Autodesk Inventor part; units mm, degrees
ref_plane "YZ Plane" through (0, 0, 0) normal (1, 0, 0) x (0, 1, 0)
ref_plane "XZ Plane" through (0, 0, 0) normal (0, 1, 0) x (-1, 0, 0)
ref_plane "XY Plane" through (0, 0, 0) normal (0, 0, 1) x (1, 0, 0)
sketch "Sketch1" plane through (0, 0, 0) normal (0, 1, 0) x (-1, 0, 0)
  circle A0 centre (0, 0) radius 285
  circle A1 centre (0, 0) radius 295
  circle A2 centre (0, 0) radius 275
  circle A3 centre (0, 0) radius 305
  line L0 (0, 0) -> (300.3664, -52.9627)
  line L1 (0, 0) -> (305, 0)
  point P0 (275, 0)
  point P1 (270.8221, -47.7532)
  dimension "d1" = 590
  dimension "d5" = 10
  dimension "d6" = 10
  dimension "d7" = 10
  dimension "d8" = 10
extrude "Extrusion1" add sketch "Sketch1" along normal blind 10 contours L1 A1 L0 A0 | A0 L0 A2 L1 | L1 A3 L0 A1 picked at (291.5003, -5.7176) picked at (281.3509, -10.8537) picked at (297.9408, -46.5324)
sketch "Sketch2" plane through (0, 10, 0) normal (0, 1, 0) x (1, 0, 0)
  arc A0 (-270.8221, 47.7532) -> (-275, 0) centre (0, 0) ccw
  line L0 (-270.8221, 47.7532) -> (-300.3664, 52.9627)
  arc A1 (-300.3664, 52.9627) -> (-305, 0) centre (0, 0) ccw
  line L1 (-305, 0) -> (-275, 0)
  circle A2 centre (0, 0) radius 295
  circle A3 centre (0, 0) radius 285
  point P0 (-285, 0)
  point P1 (-280.6702, 49.4897)
  point P2 (-290.5183, 51.2262)
  point P3 (-295, 0)
  dimension "d11" = 10
  dimension "d12" = 590
extrude "Extrusion2" add sketch "Sketch2" along normal blind 5 contours A3 L1 A2 L0 picked at (-291.3396, 11.2413)
sketch "Sketch3" plane through (0, 15, 0) normal (0, 1, 0) x (1, 0, 0)
  line L0 (-290.5183, 51.2262) -> (-300.3664, 52.9627)
  arc A0 (-300.3664, 52.9627) -> (-305, 0) centre (0, 0) ccw
  line L1 (-305, 0) -> (-295, 0)
  line L2 (-280.6702, 49.4897) -> (-290.5183, 51.2262)
  arc A1 (-290.5183, 51.2262) -> (-295, 0) centre (0, 0) ccw
  line L3 (-295, 0) -> (-285, 0)
  arc A2 (-280.6702, 49.4897) -> (-285, 0) centre (0, 0) ccw
  line L4 (-285, 0) -> (-275, 0)
  arc A3 (-270.8221, 47.7532) -> (-275, 0) centre (0, 0) ccw
  line L5 (-270.8221, 47.7532) -> (-280.6702, 49.4897)
  circle A4 centre (0, 0) radius 305
  circle A5 centre (0, 0) radius 275
  line L6 (0, 0) -> (-304.7097, -13.3039)
  line L7 (0, 0) -> (-297.7703, 66.0141)
  arc A6 (-300.3664, 52.9627) -> (-305, 0) centre (0, 0) ccw
  arc A7 (-270.8221, 47.7532) -> (-275, 0) centre (0, 0) ccw
  arc A8 (-290.5183, 51.2262) -> (-295, 0) centre (0, 0) ccw
  line L8 (-290.5183, 51.2262) -> (-300.3664, 52.9627)
  line L9 (-305, 0) -> (-295, 0)
  arc A9 (-280.6702, 49.4897) -> (-285, 0) centre (0, 0) ccw
  arc A10 (-290.5183, 51.2262) -> (-295, 0) centre (0, 0) ccw
  arc A11 (-280.6702, 49.4897) -> (-285, 0) centre (0, 0) ccw
  line L10 (-285, 0) -> (-275, 0)
  line L11 (-270.8221, 47.7532) -> (-280.6702, 49.4897)
  point P0 (-270.8221, 47.7532)
  point P1 (-268.4814, 59.5209)
  point P2 (-305, 0)
  point P3 (-274.7383, -11.9953)
  point P4 (-305, 0)
  point P5 (-300.3664, 52.9627)
  point P6 (-305, 0)
  point P7 (-270.8221, 47.7532)
  dimension "d23" = 2.5
  dimension "d24" = 2.5
extrude "Extrusion3" add sketch "Sketch3" along normal blind 10 contours A1 L1 A0 L0 | L0 A4 L7 A5 L5 L2 | L2 A2 L3 A1 | L5 A3 L4 A2 | L3 L4 A5 L6 A4 L1
sketch "Sketch4" plane through (0, 0, 0) normal (0, -1, 0) x (1, 0, 0)
  arc A0 (-275, 0) -> (-270.8221, -47.7532) centre (0, 0) ccw
  line L0 (-305, 0) -> (-275, 0)
  arc A1 (-305, 0) -> (-300.3664, -52.9627) centre (0, 0) ccw
  line L1 (-270.8221, -47.7532) -> (-300.3664, -52.9627)
  circle A2 centre (0, 0) radius 285
  circle A3 centre (0, 0) radius 295
  point P0 (-295, 0)
  point P1 (-290.5183, -51.2262)
  point P2 (-280.6702, -49.4897)
  point P3 (-285, 0)
  dimension "d17" = 10
  dimension "d18" = 590
extrude "Extrusion4" add sketch "Sketch4" along normal blind 30 contours A2 L1 A3 L0 picked at (-291.3396, -11.2413)
sketch "Sketch5" plane through (0, -30, 0) normal (0, -1, 0) x (1, 0, 0)
  arc A0 (-295, 0) -> (-290.5183, -51.2262) centre (0, 0) ccw
  line L0 (-290.5183, -51.2262) -> (-280.6702, -49.4897)
  arc A1 (-285, 0) -> (-280.6702, -49.4897) centre (0, 0) ccw
  line L1 (-285, 0) -> (-295, 0)
  arc A2 (-295, 0) -> (-290.5183, -51.2262) centre (0, 0) ccw
  line L2 (-305, 0) -> (-295, 0)
  arc A3 (-305, 0) -> (-300.3664, -52.9627) centre (0, 0) ccw
  line L3 (-290.5183, -51.2262) -> (-300.3664, -52.9627)
  line L4 (-270.8221, -47.7532) -> (-280.6702, -49.4897)
  arc A4 (-275, 0) -> (-270.8221, -47.7532) centre (0, 0) ccw
  line L5 (-285, 0) -> (-275, 0)
  arc A5 (-305, 0) -> (-300.3664, -52.9627) centre (0, 0) ccw
  arc A6 (-275, 0) -> (-270.8221, -47.7532) centre (0, 0) ccw
  arc A7 (-285, 0) -> (-280.6702, -49.4897) centre (0, 0) ccw
  arc A8 (-295, 0) -> (-290.5183, -51.2262) centre (0, 0) ccw
  line L6 (-305, 0) -> (-295, 0)
  line L7 (-290.5183, -51.2262) -> (-300.3664, -52.9627)
  arc A9 (-285, 0) -> (-280.6702, -49.4897) centre (0, 0) ccw
  line L8 (-270.8221, -47.7532) -> (-280.6702, -49.4897)
  line L9 (-285, 0) -> (-275, 0)
  arc A10 (-295, 0) -> (-290.5183, -51.2262) centre (0, 0) ccw
  circle A11 centre (0, 0) radius 265
  line L10 (0, 0) -> (-305, 0)
  line L11 (0, 0) -> (-300.3664, -52.9627)
  point P0 (-290.5183, -51.2262)
  point P1 (-260.9741, -46.0168)
  point P2 (-265, 0)
  dimension "d25" = 30
extrude "Extrusion5" add sketch "Sketch5" along normal blind 10 contours L1 A1 L0 A0 | L5 A4 L4 A1 | L10 A11 L11 A4
properties part number "Moving Caoursel base Clip"
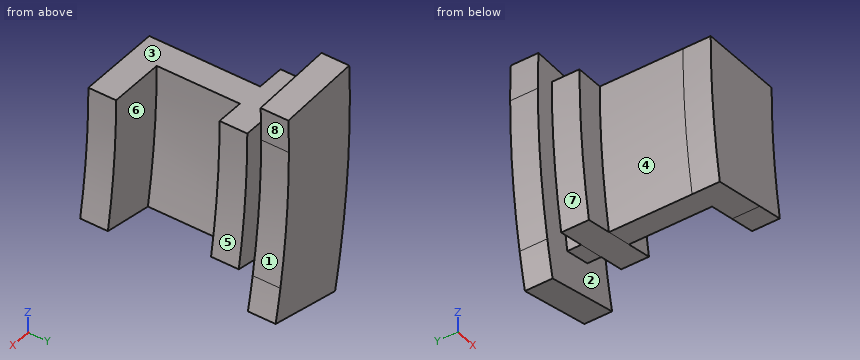
Can you work these out from the model? Positions are in its coordinate system, mm. Face numbers are marked on the shaded views. A direction names the side the tool comes from. Give positions to 0.01 mm unless a question says otherwise; leave off trailing zeros. Loops run counter-clockwise (first coordinate to the right, second up) from the corner with the lowest first, then second, coordinate; pieces in that order, holes last. Notation, with made-up numbers: M 46.25,35.25 L 72.25,35.25 A23 ccw 72.25,58.25 Z; hole C 72,-15.75 d8. An arc over 180 degrees is marked long. Use one line per item in the form item = value. Start each with the question number.
(1) I want a section at C-C, the plane z = -41. Write out the boundary of the cut face in (x, y).
(2) Please list where these lines run through material, in increasing order: line 1 (Y direction, x = -279.5, z = -17.5); line 2 (Y direction, x = -299, z = -45.5); line 3 (Y direction, x = -265.5, z = -34.5).
(3) I want a section at A-A, the plane y = 16. Write out the boundary of the cut face in (x, z), and give its area (3 significant figures).
(4) On a 3-axis mill with a long thin cutter (end or side, diameter ignored), from which of +Z, -Z, +X, -X, +Y, -Y can I reach the whole of each face in a straight line? I mean the marked faces 1, 2, 3, 4 and 5. Say none if no direction works.
(5) Thinking about a two-plate mould opening in Z: for the marked faces 6, 7 and 8, which applies, released by +Z, released by -Z, zero draft, split by the parting line, or undercut?
(6) I'm going to push flat-ended pins straight in: P1, Ø3, axis at x = -288.5, y = -2, coming from the +Z side; P2, Ø10, axis at x = -274, y = 11.5, coming from the -Z side; P3, Ø2, axis at y = -33.5, z = -10, coming from the -X side. Where does each tip first touch, or does it pass through?
Worked out:
q1.outline = M -302.23,0 L -292.14,0 L -292.14,-40 L -261.81,-40 L -261.81,-30 L -282.04,-30 L -282.04,0 L -271.93,0 L -271.93,10 L -282.04,10 L -282.04,15 L -271.93,15 L -271.93,25 L -302.23,25 L -302.23,15 L -292.14,15 L -292.14,10 L -302.23,10 Z
q2.line_1 = -40 to -30, 0 to 10, 15 to 25
q2.line_2 = 0 to 10, 15 to 25
q2.line_3 = -40 to -30
q3.outline = M -305,0 A305 ccw -300.37,-52.96 A305 ccw -297.77,-66.01 L -268.48,-59.52 A275 cw -270.82,-47.75 A275.01 cw -275,0 A275 cw -274.74,12 L -304.71,13.3 A305 ccw Z
q3.area = 2,280 mm²
q4.face_1 = +X, +Y
q4.face_2 = none
q4.face_3 = +Z, +X, -X, -Y
q4.face_4 = -Z, -X, -Y
q4.face_5 = +Z, +X, +Y
q5.face_6 = zero draft
q5.face_7 = released by -Z
q5.face_8 = undercut
q6.P1 = 0
q6.P2 = -61.54
q6.P3 = -294.86
